Source: CAD feature listing. Evaluate the final solid. Frame: model axes, mm. Round coordinates to 2 decimals unless told otherwise and drop trailing zeros. Order: outer loops, then holes, each group sorted by start corner. A loop starts at its lowest first (then second) coordinate and runs counter-clockwise, first axis right, second up. Notation, with made-up numbers: M -24,-35 L -9,-35 A31 cw -9,-5 Z; hole C 69,59 d6. An arc over 180 degrees is marked long. Answer as CSV lines item,"result". Start each with the question number.
Item 1: Line query: line 1 (X direction, y = -16, z = 3.5); line 2 (Y direction, x = 31.75, z = 1.75); line 3 (Y direction, x = 7, z = 1.5). Output: solid intervals per line, ascending. Write a range as [from, to].
Item 2: Section query A-A on x = 31.75. Return the cut outline in (y, z).
Item 3: First-contact query: P1, Ø5.5, axis at x = 55.22, y = -64.36, coming from the +Z side; P2, Ø5.5, axis at x = 31.75, y = -40.894, coming from the +Z side (1 decimal). Flat tips, straight axial feed; report the tip coordinate or a pass-through.
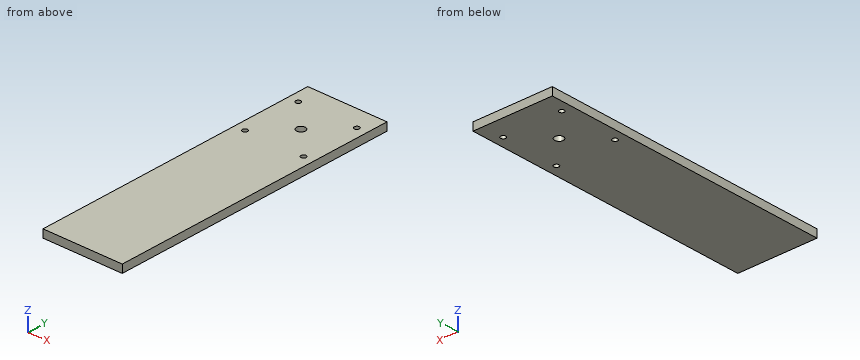
from build123d import *

# Parameters (mm, degrees)
SKETCH1_W                  = 63.5
SKETCH1_H                  = 233.172
SKETCH1_R                  = 3.4925
BOSS_EXTRUDE1_DEPTH        = 6.35
F_10_32_TAPPED_HOLE1_D     = 4.0386
F_10_32_TAPPED_HOLE1_DEPTH = 6.35


with BuildPart() as part:
    # Sketch1 → Boss-Extrude1 (new body)
    with BuildSketch(Plane.XY):
        with Locations((31.75, -116.586)):
            Rectangle(SKETCH1_W, SKETCH1_H)
        with Locations((31.75, -40.894)):
            Circle(SKETCH1_R, mode=Mode.SUBTRACT)
    extrude(amount=BOSS_EXTRUDE1_DEPTH)

    # #10-32 Tapped Hole1
    with Locations(Plane.XY.offset(6.35)):
        with Locations((8.2804, -17.4244), (55.2196, -17.4244), (55.2196, -64.3636), (8.2804, -64.3636)):
            Hole(F_10_32_TAPPED_HOLE1_D / 2, depth=F_10_32_TAPPED_HOLE1_DEPTH)


solid = part.part
Results:
1,line 1,"[0, 6.85], [9.71, 53.79], [56.65, 63.5]"
1,line 2,"[-233.17, -44.39], [-37.4, 0]"
1,line 3,"[-233.17, -65.93], [-62.8, -18.99], [-15.86, 0]"
2,outline,"M -233.17,0 L -44.39,0 L -44.39,6.35 L -233.17,6.35 Z; M -37.4,0 L 0,0 L 0,6.35 L -37.4,6.35 Z"
3,P1,"z = 6.35"
3,P2,"through"
